Read the model definition and answer for the solid it produces. Units are mm, in the model's axes. A direction names the side the tool comes from. Round coordinates to 2 decimals unless told otherwise and drop trailing zeros. Loops run counter-clockwise (first coordinate to the right, second up) from the corner with the lowest first, then second, coordinate; pieces in that order, holes last. Notation, with made-up numbers: (-8.75, 73.25) - (14.25, 73.25) arc R31 cw to (14.25, 111.25) - close; hole circle Ø2 at (20, 51). An arc over 180 degrees is marked (long way). Use CSV: the item, a comma, the result in double quotes. Start each with the question number.
1. Find section A-A (x = 0). Give the vertices of the cut face in (y, z).
2. Given pin 1 Ø6 at (y, z) = (27.5, 12) entering from -X; pin 2 Ø2 at (x, y) = (7, 8.5) entering from +Z; pin 3 Ø3 at (x, y) = (-1, 21) entering from +Z, each flat-ended and moving along its own axis, determine where each tip first touches the part or whether it passes through.
3. Find section D-D (z = 14). Give the vertices of the cut face in (x, y).
4. A tool of negligible diameter and unlimited length cuts with its end or side. For faces 1 (the flat face through (14, 37, -6)), 2 (the flat face through (6, 0, 0)), 3 (the flat face through (5.15, 18, 0)), 4 (the flat face through (-5.643, 38.607, 0.086)), from which of +Z, -Z, +X, -X, +Y, -Y can it reach the whole face along a straight path? Write none if from no direction.
5. Find section C-C (y = 32). Give the vertices of the cut face in (x, z).
6. Find section B-B (z = 0). Give the vertices of the cut face in (x, y).
7. Consider line 1 along X through (y, z) = (27, 0); line 2 along Z through (x, y) = (-0.5, 12); line 3 along Y through (x, z) = (-16, 1.5). Determine where each line is inside the solid, lowest interval first.
8. Determine the mould class of faces 5 (the flat face through (-5.15, 18, 0)), 6 (the flat face through (8, 40, 0)), 7 (the cylindrical face through (8.767, 38.521, 16.856)) for opening direction Z: +Z half, -Z half, draft (parallel to the pull), parting line (faces both ways), or undercut.
from build123d import *

# Parameters (mm, degrees)
SKETCH_1_R          = 15
SKETCH_1_W          = 10.3
SKETCH_1_H          = 10.3
EXTRUDE_1_DEPTH     = 40
SKETCH1_R           = 19
SKETCH1_W           = 10.3
SKETCH1_H           = 10.3
BOSS_EXTRUDE1_DEPTH = 3
CHAMFER1_SIZE       = 1
CHAMFER1_SIZE2      = 2.747477419


with BuildPart() as part:
    # Эскиз1 → Бобышка-Вытянуть1 (new body)
    with BuildSketch(Plane(origin=(0, 0, 0), x_dir=(1, 0, 0), z_dir=(0, 1, 0))):
        Circle(SKETCH_1_R)
        Rectangle(SKETCH_1_W, SKETCH_1_H, mode=Mode.SUBTRACT)
    extrude(amount=EXTRUDE_1_DEPTH)

    # Sketch1 → Boss-Extrude1 (add)
    with BuildSketch(Plane(origin=(0, 40, 0), x_dir=(1, 0, 0), z_dir=(0, 1, 0))):
        Circle(SKETCH1_R)
        Rectangle(SKETCH1_W, SKETCH1_H, mode=Mode.SUBTRACT)
    extrude(amount=-BOSS_EXTRUDE1_DEPTH)

    # Chamfer1
    chamfer1_edges = [part.edges().sort_by_distance(p)[0] for p in [
        (0, 40, -5.15),
        (-5.15, 40, 0),
        (0, 40, 5.15),
        (5.15, 40, 0),
    ]]
    chamfer1_side = [part.faces().sort_by_distance(p)[0] for p in [
        (-18.462598846, 40, 0),
    ]]
    chamfer(chamfer1_edges, length=CHAMFER1_SIZE, length2=CHAMFER1_SIZE2, reference=chamfer1_side[0])


solid = part.part
Filled sheet:
1,outline,"(0, -15) - (37, -15) - (37, -19) - (40, -19) - (40, -6.15) - (37.25, -5.15) - (0, -5.15) - close; (0, 5.15) - (37.25, 5.15) - (40, 6.15) - (40, 19) - (37, 19) - (37, 15) - (0, 15) - close"
2,pin 1,"stops at x = -12"
2,pin 2,"stops at z = 13.75"
2,pin 3,"stops at z = 15"
3,outline,"(-12.85, 37) - (-5.39, 37) - (-5.39, 0) - (5.39, 0) - (5.39, 37) - (12.85, 37) - (12.85, 40) - (-12.85, 40) - close"
4,face 1,"-Y"
4,face 2,"+Z, -Z, +X, -X, -Y"
4,face 3,"+Y, -Y"
4,face 4,"+Y"
5,outline,"circle Ø30 at (0, 0); hole (-5.15, -5.15) - (5.15, -5.15) - (5.15, 5.15) - (-5.15, 5.15) - close"
6,outline,"(-19, 37) - (-15, 37) - (-15, 0) - (-5.15, 0) - (-5.15, 37.25) - (-6.15, 40) - (-19, 40) - close; (5.15, 0) - (15, 0) - (15, 37) - (19, 37) - (19, 40) - (6.15, 40) - (5.15, 37.25) - close"
7,line 1,"x = -15 to -5.15, 5.15 to 15"
7,line 2,"z = -14.99 to -5.15, 5.15 to 14.99"
7,line 3,"y = 37 to 40"
8,face 5,"undercut"
8,face 6,"draft"
8,face 7,"parting line"
